The listing builds one solid part. Answer for the finished solid, in the listing's coordinates (mm). Give positions to 0.01 mm unless a question says otherwise; leave off trailing zeros. Write each loop counter-clockwise with the first axis right and the second up, starting at its lowest first coordinate (ties: lowest second). Pieces come first, ordered by that corner, then holes. Notation, with made-up numbers: (10, -28) -> (33, -28) arc R29 ccw to (33, 7) -> close; hole circle Ø11 at (-15.5, -28). An arc over 180 degrees is marked (long way). Put each result on its own line as item: value. Start each with the question number.
1) For a pull along Y with two mould halves and no side action, classify faces 1 (the flat face through (1, 32.315, 3)), 2 (the flat face through (-1, 53, 6)), 3 (the cylindrical face through (-39.312, 34.909, 2.958)), 4 (the flat face through (1, 72.315, 3)) as released by +Y, released by -Y, zero draft, split by the parting line, or undercut.
2) Find the intervals of material crossed by line 1 along Y through (x, z) = (40.6, 2.05) (3 decimals); line 2 along X through (y, z) = (36, 4.45); line 3 along Y through (x, z) = (32, 3.65) (3 decimals), in increasing order. Write a range as from..to.
3) A cutting plane is placed at A-A (x = 40.6). Write down the section's boundary in (y, z) (3 decimals).
Autodesk Inventor part; units mm, degrees
ref_plane "YZ Plane" through (0, 0, 0) normal (1, 0, 0) x (0, 1, 0)
ref_plane "XZ Plane" through (0, 0, 0) normal (0, 1, 0) x (-1, 0, 0)
ref_plane "XY Plane" through (0, 0, 0) normal (0, 0, 1) x (1, 0, 0)
ref_plane "작업 평면1" through (0, 0, -13) normal (0, 0, 1) x (1, 0, 0)
ref_plane "작업 평면2" through (0, 0, 0) normal (0, 0, 1) x (1, 0, 0)
sketch "스케치2" plane through (0, 0, 0) normal (0, 0, 1) x (1, 0, 0)
  circle A0 centre (-40.6, 35.315) radius 1.35
  circle A1 centre (-30.7755, 35.315) radius 1.35
  line L0 (-22.2, 38.315) -> (-49.8, 38.315)
  line L1 (-49.8, 38.315) -> (-49.8, 32.315)
  line L2 (-22.2, 32.315) -> (-49.8, 32.315)
  line L3 (-22.2, 38.315) -> (-22.2, 32.315)
  circle A2 centre (40.6, 35.315) radius 1.35
  circle A3 centre (30.7755, 35.315) radius 1.35
  line L4 (22.2, 38.315) -> (49.8, 38.315)
  line L5 (22.2, 38.315) -> (22.2, 32.315)
  line L6 (22.2, 32.315) -> (49.8, 32.315)
  line L7 (49.8, 38.315) -> (49.8, 32.315)
  line L8 (-49.8, 32.315) -> (49.8, 32.315)
  line L9 (49.8, 32.315) -> (49.8, 72.315)
  line L10 (49.8, 72.315) -> (-49.8, 72.315)
  line L11 (-49.8, 72.315) -> (-49.8, 32.315)
  point P0 (0, 0)
  dimension "d3" = 40
extrude "돌출2" add sketch "스케치2" along normal blind 6
sketch "스케치3" plane through (0, 0, 6) normal (0, 0, 1) x (1, 0, 0)
  line L0 (-49.8, 32.315) -> (49.8, 32.315)
  line L1 (49.8, 32.315) -> (49.8, 72.315)
  line L2 (49.8, 72.315) -> (-49.8, 72.315)
  line L3 (-49.8, 72.315) -> (-49.8, 32.315)
  circle A0 centre (40.6, 35.315) radius 1.35
  circle A1 centre (30.7755, 35.315) radius 1.35
  circle A2 centre (-40.6, 35.315) radius 1.35
  circle A3 centre (-30.7755, 35.315) radius 1.35
  line L4 (46.167, 64.315) -> (-44.5, 64.315)
  line L5 (49.5, 64.315) -> (46.167, 64.315)
  line L6 (-51.5, 64.315) -> (-44.5, 64.315)
  line L7 (-49.8, 72.315) -> (-49.8, 66.315)
  line L8 (-49.8, 66.315) -> (49.8, 66.315)
  line L9 (49.8, 66.315) -> (49.8, 72.315)
  line L10 (49.8, 72.315) -> (-49.8, 72.315)
  line L11 (49.8, 72.315) -> (16.6, 72.315)
  line L12 (16.6, 72.315) -> (-16.6, 72.315)
  line L13 (-16.6, 72.315) -> (-16.6, 66.315)
  line L14 (16.6, 72.315) -> (16.6, 66.315)
  circle A4 centre (16.6, 69.315) radius 1.35
  circle A5 centre (-16.6, 69.315) radius 1.35
  point P0 (0, 0)
  point P1 (0, 72.315)
  dimension "d6" = 6
  dimension "d7" = 33.2
  dimension "d8" = 33.2
  dimension "d9" = 2.7
  dimension "d10" = 2.7
extrude "돌출3" cut sketch "스케치3" against normal blind 6 contours A4 L14 | L14 A4 | A5 L13 | L13 A5
properties part number "_battery_adt"
Reply:
1. face 1: released by -Y
1. face 2: zero draft
1. face 3: undercut
1. face 4: released by +Y
2. line 1: y = 32.315..33.965, 36.665..72.315
2. line 2: x = -49.8..-41.76, -39.44..-31.94, -29.61..29.61, 31.94..39.44, 41.76..49.8
2. line 3: y = 32.315..34.747, 35.883..72.315
3. outline: (32.315, 0) -> (33.965, 0) -> (33.965, 6) -> (32.315, 6) -> close; (36.665, 0) -> (72.315, 0) -> (72.315, 6) -> (36.665, 6) -> close
